Here's how the part is built. I have some questions about the finished solid (model axes, mm). Round coordinates to 2 decimals unless told otherwise and drop trailing zeros. Loops run counter-clockwise (first coordinate to the right, second up) from the corner with the lowest first, then second, coordinate; pieces in that order, holes last. Notation, with made-up numbers: M -4,58 L 18,58 A26 ccw 18,97 Z; hole C 7,7.5 d9. An arc over 180 degrees is marked long. Use a Markdown table: item, result.
from build123d import *

# Parameters (mm, degrees)
SKETCH1_W               = 38.1
SKETCH1_H               = 38.1
BOSS_EXTRUDE1_DEPTH     = 770.128
CUT_EXTRUDE1_DEPTH      = 772.305159379
CUT_EXTRUDE2_DEPTH      = 772.305159379
CUT_EXTRUDE2_DEPTH_BACK = 772.305159379


with BuildPart() as part:
    # Sketch1 → Boss-Extrude1 (new body)
    with BuildSketch(Plane(origin=(0, 0, 0), x_dir=(0, 0, -1), z_dir=(1, 0, 0))):
        Rectangle(SKETCH1_W, SKETCH1_H)
    extrude(amount=BOSS_EXTRUDE1_DEPTH)

    # Sketch2 → Cut-Extrude1 (cut, through all)
    with BuildSketch(Plane.XY.offset(19.05)):
        Polygon((770.128, -19.05), (749.869870654, 19.05), (770.128, 19.05), align=None)
    extrude(amount=-CUT_EXTRUDE1_DEPTH, mode=Mode.SUBTRACT)

    # Sketch3 → Cut-Extrude2 (cut, two sides: drawn at the far end of the back side and taken through both)
    with BuildSketch(Plane.XY.offset(19.05).offset(-CUT_EXTRUDE2_DEPTH_BACK)):
        Polygon((0, -19.05), (22.426868859, -7.125422305), (-1.422286531, 37.728315412), (-23.84915539, 25.803737717), align=None)
    extrude(amount=CUT_EXTRUDE2_DEPTH + CUT_EXTRUDE2_DEPTH_BACK, mode=Mode.SUBTRACT)


solid = part.part
1. I need wall thicknesses on probe 1 along X at (y, z) = (-7.5, 1); probe 2 along X at (y, z) = (11.5, -13). Which ranges of each line are inside material? Lowest first, please. Write a range as from..to.
Answer sheet:
| item | result |
|---|---|
| probe 1 | 21.72..763.99 |
| probe 2 | 12.52..753.88 |
2. Imagine slicing it at B-B, the plane y = 3. Write out the boundary of the cut face in (x, z).
Answer sheet:
| item | result |
|---|---|
| outline | M 17.04,-19.05 L 758.4,-19.05 L 758.4,19.05 L 17.04,19.05 Z |
3. For pin 1 Ø10 at (y, z) = (-10.5, 6) entering from +X; pin 2 Ø3 at (y, z) = (5.5, -1) entering from +X; pin 3 Ø8 at (y, z) = (-15, 6.5) entering from -X, each with a flat end and sliding along its axis, tell me the tip position at first contact or that it passes through.
Answer sheet:
| item | result |
|---|---|
| pin 1 | x = 768.24 |
| pin 2 | x = 757.87 |
| pin 3 | x = 0.09 |
4. Imagine slicing it at A-A, the plane z = 8.5. Write out the boundary of the cut face in (x, y), then the cut area to 3 significant figures.
Answer sheet:
| item | result |
|---|---|
| outline | M 0,-19.05 L 770.13,-19.05 L 749.87,19.05 L 8.51,19.05 L 22.43,-7.13 Z |
| area | 28,400 mm2 |
5. We'd pull the mould along Y, two halves only. Please class faces 1 (the face through (380, -19.05, 0)), 2 (the face through (15.565, 5.779, -0.267)), 3 (the face through (11.06, -13.17, -0.27)), 4 (the face through (380, 0, 19.05)): +Y half, -Y half, draft (parallel to the pull), parting line (faces both ways), or undercut.
Answer sheet:
| item | result |
|---|---|
| face 1 | -Y half |
| face 2 | undercut |
| face 3 | undercut |
| face 4 | draft |
